Design review of the part shown in the three views and the two pictorial views. Dimensions are in mm from the part's minimum x, y and z. A direction names the side the tool comes from. Coordinates: 2 decimals unless noted, no trailing zeros. Loops run counter-clockwise (first coordinate to the right, second up) from the corner with the lowest first, then second, coordinate; pieces in that order, holes last. Notation, with made-up numbers: (42, -22) -> (59, -22) arc R13 cw to (59, -1) -> close; hole circle Ø2 at (5, 47.5). An arc over 180 degrees is marked (long way). Use a Markdown table: item, result. Add a question column.
Q1. Clearance check with flat-ended pins moving along their axes: pin 1 Ø3 at (x, y) = (11.5, 80.5) entering from +Z; pin 2 Ø20 at (x, y) = (41.8, 45) entering from +Z. State where each tip first meets the part, or that it passes through.
Q2. Take a section at A-A on x = 69.8. Write out the cut boundary in (y, z).
Q3. For probe 1 along Y at (x, z) = (13.8, 1.5); probe 2 along Y at (x, z) = (41, 5.75); probe 3 along Y at (x, z) = (13.8, 10.75), list the stretches that pass through material, from the lowest coordinate up.
Q4. Take a section at B-B on y = 13. Write out the cut boundary in (x, z).
Q5. For the marked faces 4, 5 and 6, list the 3-axis set-ups (+Z, -Z, +X, -X, +Y, -Y) from which the entire face can be reached by the end or side of a thin tool; tool diameter is ignored.
Q6. Draft analysis for pull direction X (two halves, no side actions). For the marked faces 1, 2 and 3, state which applies: pulls with the +X half, pulls with the -X half, needs draft (parallel to the pull), parting line crosses it, or undercut.
Q7. Take a section at D-D on z = 2.25. Write out the cut boundary in (x, y).
Q8. Take a section at C-C on x = 41.8. Write out the cut boundary in (y, z).
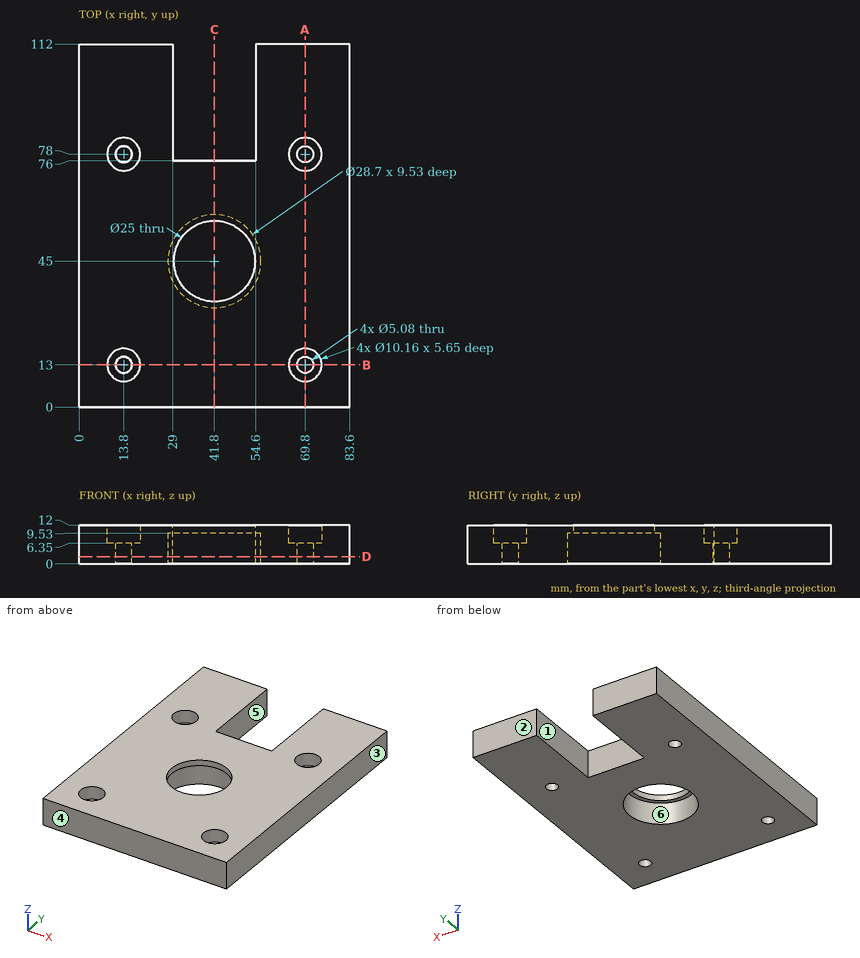
Answer list:
| question | item | result |
|---|---|---|
| 1 | pin 1 | z = 6.35 |
| 1 | pin 2 | through |
| 2 | outline | (0, 0) -> (10.46, 0) -> (10.46, 6.35) -> (7.92, 6.35) -> (7.92, 12) -> (0, 12) -> close; (15.54, 0) -> (75.46, 0) -> (75.46, 6.35) -> (72.92, 6.35) -> (72.92, 12) -> (18.08, 12) -> (18.08, 6.35) -> (15.54, 6.35) -> close; (80.54, 0) -> (112, 0) -> (112, 12) -> (83.08, 12) -> (83.08, 6.35) -> (80.54, 6.35) -> close |
| 3 | probe 1 | 0 to 10.46, 15.54 to 75.46, 80.54 to 112 |
| 3 | probe 2 | 0 to 30.67, 59.33 to 76 |
| 3 | probe 3 | 0 to 7.92, 18.08 to 72.92, 83.08 to 112 |
| 4 | outline | (0, 0) -> (11.26, 0) -> (11.26, 6.35) -> (8.72, 6.35) -> (8.72, 12) -> (0, 12) -> close; (16.34, 0) -> (67.26, 0) -> (67.26, 6.35) -> (64.72, 6.35) -> (64.72, 12) -> (18.88, 12) -> (18.88, 6.35) -> (16.34, 6.35) -> close; (72.34, 0) -> (83.6, 0) -> (83.6, 12) -> (74.88, 12) -> (74.88, 6.35) -> (72.34, 6.35) -> close |
| 5 | face 4 | +Z, -Z, +X, -X, -Y |
| 5 | face 5 | +Z, -Z, +Y |
| 5 | face 6 | -Z |
| 6 | face 1 | undercut |
| 6 | face 2 | needs draft |
| 6 | face 3 | pulls with the +X half |
| 7 | outline | (0, 0) -> (83.6, 0) -> (83.6, 112) -> (54.6, 112) -> (54.6, 76) -> (29, 76) -> (29, 112) -> (0, 112) -> close; hole circle Ø5.08 at (13.8, 13); hole circle Ø5.08 at (13.8, 78); hole circle Ø28.7 at (41.8, 45); hole circle Ø5.08 at (69.8, 13); hole circle Ø5.08 at (69.8, 78) |
| 8 | outline | (0, 0) -> (30.65, 0) -> (30.65, 9.53) -> (32.5, 9.53) -> (32.5, 12) -> (0, 12) -> close; (57.5, 9.53) -> (59.35, 9.53) -> (59.35, 0) -> (76, 0) -> (76, 12) -> (57.5, 12) -> close |
